```python
from build123d import *

# Parameters (mm, degrees)
BOSS_EXTRUDE1_DEPTH = 100
SKETCH2_R           = 2
CUT_EXTRUDE1_DEPTH  = 100
SKETCH3_W           = 5
SKETCH3_H           = 12
BOSS_EXTRUDE2_DEPTH = 2


with BuildPart() as part:
    # Sketch1 → Boss-Extrude1 (new body)
    with BuildSketch(Plane.XY):
        Polygon((0, 0), (7, 0), (7, 12), (15, 12), (15, 9), (10, 9), (10, -3), (0, -3), align=None)
    extrude(amount=BOSS_EXTRUDE1_DEPTH)

    # Sketch2 → Cut-Extrude1 (cut)
    with BuildSketch(Plane(origin=(0, 0, 0), x_dir=(1, 0, 0), z_dir=(0, 1, 0))):
        with Locations((3.5, -10)):
            Circle(SKETCH2_R)
        with Locations((3.5, -90)):
            Circle(SKETCH2_R)
        with Locations((3.5, -50)):
            Circle(SKETCH2_R)
    extrude(amount=-CUT_EXTRUDE1_DEPTH, mode=Mode.SUBTRACT)

    # Sketch3 → Boss-Extrude2 (add)
    with BuildSketch(Plane(origin=(0, 0, 0), x_dir=(-1, 0, 0), z_dir=(0, 0, -1))):
        with Locations((-12.5, 3)):
            Rectangle(SKETCH3_W, SKETCH3_H)
    extrude(amount=-BOSS_EXTRUDE2_DEPTH)


solid = part.part
```
Model file for the job. Use its own axes, mm. A direction names the side the tool comes from. Round coordinates to 2 decimals unless told otherwise and drop trailing zeros. Loops run counter-clockwise (first coordinate to the right, second up) from the corner with the lowest first, then second, coordinate; pieces in that order, holes last. Notation, with made-up numbers: M 44,-37 L 99,-37 A32 cw 99,1 Z; hole C 53.5,40 d2. An arc over 180 degrees is marked long. Put each result on its own line as item: value. Start each with the question number.
Item 1: Drill centre lines: line 1 along X through (y, z) = (-1.35, 10); line 2 along Z through (x, y) = (3.5, -1); line 3 along X through (y, z) = (-2.5, 93.5). Where is each one in solid material? Low to high.
Item 2: Cut at C-C (z = 34.5). List the corners of the cut face in (x, y).
Item 3: Cut at A-A (z = 90). List the corners of the cut face in (x, y).
Item 4: 3-axis set-ups, long thin cutter, end or side, ignore diameter. For faces 5 (the face through (13, 3, 2)), 6 (the face through (9, 3, 0)), 7 (the face through (7, 6, 49)): which of +Z, -Z, +X, -X, +Y, -Y reach the whole face in a straight line?
Item 5: Cut at D-D (x = 13.25). List the corners of the cut face in (y, z).
Item 6: Mould opens along X. For faces 1 (the face through (3.24, -1.479, 88.017)), 2 (the face through (10, 3, 50)), 3 (the face through (6, -3, 49)), 4 (the face through (3.066, -1.479, 51.952)) say: released by +X, released by -X, zero draft, split by the parting line, or undercut.
Item 7: Cut at B-B (x = 3.5). List the corners of the cut face in (y, z), then the cut area to 3 significant figures.
Item 8: Drop flat-ended pins along their axis: P1, Ø2, axis at y = 2, z = 60.5, coming from the +X side; P2, Ø1.5, axis at x = 13.5, z = 32.5, coming from the -Y side. Give the stop position or say it passes through.
Answer block:
1. line 1: 0 to 1.5, 5.5 to 10
1. line 2: 0 to 8, 12 to 48, 52 to 88, 92 to 100
1. line 3: 0 to 10
2. outline: M 0,-3 L 10,-3 L 10,9 L 15,9 L 15,12 L 7,12 L 7,0 L 0,0 Z
3. outline: M 0,-3 L 1.5,-3 L 1.5,0 L 0,0 Z; M 5.5,-3 L 10,-3 L 10,9 L 15,9 L 15,12 L 7,12 L 7,0 L 5.5,0 Z
4. face 5: +Z, +X, -Y
4. face 6: -Z, +X, -X, +Y, -Y
4. face 7: +Z, -Z, -X, +Y
5. outline: M -3,0 L 12,0 L 12,100 L 9,100 L 9,2 L -3,2 Z
6. face 1: undercut
6. face 2: released by +X
6. face 3: zero draft
6. face 4: undercut
7. outline: M -3,0 L 0,0 L 0,8 L -3,8 Z; M -3,12 L 0,12 L 0,48 L -3,48 Z; M -3,52 L 0,52 L 0,88 L -3,88 Z; M -3,92 L 0,92 L 0,100 L -3,100 Z
7. area: 264 mm2
8. P1: x = 10
8. P2: y = 9
